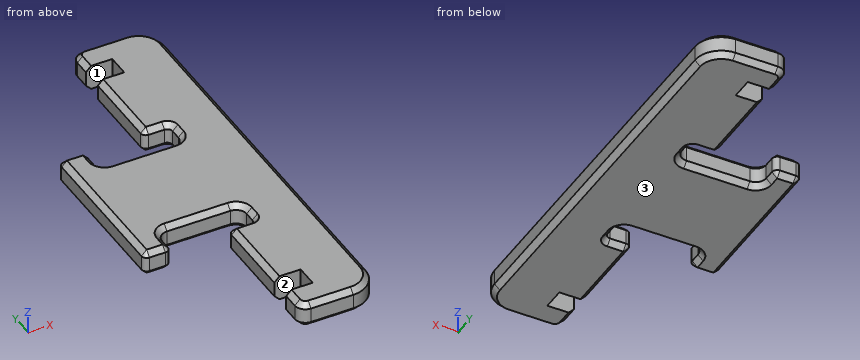
Autodesk Fusion 360 part; units mm, degrees
sketch "Sketch1" plane through (0, 0, 0) normal (0, 0, 1) x (1, 0, 0)
  line L0 (7.5, -40.2) -> (-7.5, -40.2)
  line L1 (-7.5, -40.2) -> (-7.5, 40.2)
  line L2 (-7.5, 40.2) -> (7.5, 40.2)
  line L3 (7.5, 40.2) -> (7.5, -40.2)
  line L4 (7.5, -40.2) -> (-7.5, 40.2) construction
  line L5 (-7.5, -40.2) -> (7.5, 40.2) construction
  line L6 (-7.5, 35.2) -> (-2.5, 35.2)
  line L7 (-2.5, 35.2) -> (-2.5, 31)
  line L8 (-2.5, 31) -> (-7.5, 31)
  line L9 (-7.5, 31) -> (-7.5, 35.2)
  line L10 (-7.5, -31) -> (-2.5, -31)
  line L11 (-2.5, -31) -> (-2.5, -35.2)
  line L12 (-2.5, -35.2) -> (-7.5, -35.2)
  line L13 (-7.5, -35.2) -> (-7.5, -31)
  line L14 (-2.5, 10) -> (-18.5, 10)
  line L15 (-18.5, 10) -> (-18.5, -10)
  line L16 (-18.5, -10) -> (-2.5, -10)
  line L17 (-2.5, -10) -> (-2.5, 10)
  line L18 (-23.5, 15) -> (-18.5, 15)
  line L19 (-18.5, 15) -> (-18.5, -15)
  line L20 (-18.5, -15) -> (-23.5, -15)
  line L21 (-23.5, -15) -> (-23.5, 15)
  line L22 (-2.5, -10) -> (-2.5, -15)
  line L23 (-2.5, -15) -> (-7.5, -15)
  line L24 (-2.5, 10) -> (-2.5, 15)
  line L25 (-2.5, 15) -> (-7.5, 15)
  dimension "d1" = 80.4
  dimension "d2" = 15
  dimension "d3" = 5
  dimension "d4" = 4.2
  dimension "d5" = 5
  dimension "d6" = 4.2
  dimension "d7" = 5
  dimension "d8" = 5
  dimension "d9" = 16
  dimension "d10" = 5
  dimension "d11" = 5
  dimension "d12" = 5
  dimension "d13" = 30
  dimension "d14" = 5
  dimension "d15" = 20
  dimension "d16" = 10
  dimension "d26" = 5
  dimension "d27" = 5
extrude "Extrude1" add sketch "Sketch1" along normal blind 4.8 contours L0 L1 L2 L3 L6 L7 L8 L10 L11 L12 L17 L22 L23 L24 L25 | L1 L14 L15 L16 L19 | L1 L14 L16 L17 | L15 L18 L19 L20 L21
fillet "Fillet1" radius 5 2 edges at (7.5, 40.2, 2.4) (7.5, -40.2, 2.4)
fillet "Fillet1" radius 2 6 edges at (-18.5, 10, 2.4) (-18.5, -10, 2.4) (-7.5, 40.2, 2.4) (-7.5, -40.2, 2.4) (-2.5, -10, 2.4) (-2.5, 10, 2.4)
fillet "Fillet1" radius 1 8 edges at (-18.5, 15, 2.4) (-23.5, 15, 2.4) (-18.5, -15, 2.4) (-23.5, -15, 2.4) (-2.5, 15, 2.4) (-7.5, 15, 2.4) (-2.5, -15, 2.4) (-7.5, -15, 2.4)
chamfer "Chamfer1" distance 1 angle 45 28 edges at (-10.5, 10, 4.8) (-10.5, -10, 4.8) (-10.5, -10, 0) (-10.5, 10, 0) (7.5, 0, 4.8) (7.5, 0, 0) (-18.5, -12.5, 4.8) (-18.5, -12.5, 0) (-21, -15, 4.8) (-21, -15, 0) (-23.5, 0, 4.8) (-7.5, -23, 4.8) (-7.5, -23, 0) (-7.5, -37.7, 0) (0, -40.2, 0) (0, -40.2, 4.8) (0, 40.2, 4.8) (-7.5, 37.7, 4.8) (-7.5, 37.7, 0) (-7.5, 23, 4.8) (-7.5, 23, 0) (-7.5, -37.7, 4.8) (-23.5, 0, 0) (-21, 15, 0) (0, 40.2, 0) (-18.5, 12.5, 0) (-21, 15, 4.8) (-18.5, 12.5, 4.8)
equation "d12 = d11"
equation "d16 = d15 / 2"
equation "d26 = d14"
equation "d27 = d26"
The listing builds one solid part. Answer for the finished solid, in the listing's coordinates (mm). Face numbers are marked on the shaded views. Give positions to 0.01 mm unless a question says otherwise; leave off trailing zeros. Loops run counter-clockwise (first coordinate to the right, second up) from the corner with the lowest first, then second, coordinate; pieces in that order, holes last. Notation, with made-up numbers: (45, -0.75) - (57, -0.75) arc R13 ccw to (57, 17.25) - close; hole circle Ø10 at (62, 21). An arc over 180 degrees is marked (long way). Write each question's results on one line, items separated by ' | '.
1. Find section B-B, the plane x = -13. Write down the section's boundary in (y, z).
Resolved:
outline: (-10, 1) - (-9, 0) - (9, 0) - (10, 1) - (10, 3.8) - (9, 4.8) - (-9, 4.8) - (-10, 3.8) - close
2. Find section A-A, the plane y = 13. Write down the section's boundary in (x, z).
Resolved:
outline: (-23.5, 1) - (-22.5, 0) - (-19.5, 0) - (-18.5, 1) - (-18.5, 3.8) - (-19.5, 4.8) - (-22.5, 4.8) - (-23.5, 3.8) - close; (-2.5, 1) - (-1.5, 0) - (6.5, 0) - (7.5, 1) - (7.5, 3.8) - (6.5, 4.8) - (-1.5, 4.8) - (-2.5, 3.8) - close
3. For a pull along Y with two mould halves and no side action, classify the marked faces 1, 2 and 3 as +Y half, -Y half, draft (parallel to the pull), parting line (faces both ways), or undercut.
Resolved:
face 1: undercut | face 2: undercut | face 3: draft
4. Find section C-C, the plane y = -18. Write down the section's boundary in (x, z).
Resolved:
outline: (-7.5, 1) - (-6.5, 0) - (6.5, 0) - (7.5, 1) - (7.5, 3.8) - (6.5, 4.8) - (-6.5, 4.8) - (-7.5, 3.8) - close
5. Consider probe 1 along Y at (x, z) = (-4, 1); probe 2 along X at (y, z) = (19, 2.25); probe 3 along X at (y, z) = (10.5, 0.65). Determine where each line is inside the solid, lowest interval first. Write a range as from..to.
Resolved:
probe 1: y = -40.2..-35.2, -31..-15, -10.06..10.06, 15..31, 35.2..40.2 | probe 2: x = -7.5..7.5 | probe 3: x = -23.15..-18.31, -2.69..7.15
6. Flat-ended cylindrical pins translate along their axes: P1, Ø1.4, axis at x = -12, z = 2.5, coming from the -Y side; P2, Ø1.4, axis at x = -20.5, z = 3, coming from the -Y side; P3, Ø1.5, axis at x = -18, z = 1, coming from the -Y side. Find the tip coordinate at first contact, or state that the pin passes through.
Resolved:
P1: stops at y = -10 | P2: stops at y = -15 | P3: stops at y = -14.66
